Build history of the part. All positions in model axes, mm. Face numbers are marked on the shaded views. A direction names the side the tool comes from. Round coordinates to 2 decimals unless told otherwise and drop trailing zeros. Loops run counter-clockwise (first coordinate to the right, second up) from the corner with the lowest first, then second, coordinate; pieces in that order, holes last. Notation, with made-up numbers: (2, 57.25) -> (29, 57.25) arc R22 ccw to (29, 95.25) -> close; hole circle Ø6 at (47, -15). An arc over 180 degrees is marked (long way). Put each result on its own line as item: value. Start each with the question number.
Item 1: Cut at C-C, the plane x = 10. List the corners of the cut face in (y, z).
Item 2: Drill centre lines: probe 1 along Z at (x, y) = (12.5, 35.5); probe 2 along Y at (x, z) = (-8.5, 21.75); probe 3 along X at (y, z) = (84.5, 17.25). Where is each one in solid material? Low to high. Write a range as [from, to].
Item 3: Flat gauge pins, fed straight in: pin 1 Ø0.9 at (x, z) = (17.5, 11) entering from +Y; pin 2 Ø6.5 at (y, z) = (1, 9) entering from -X; pin 3 Ø12 at (x, y) = (-0.5, -0.5) entering from +Z; pin 4 Ø0.9 at (x, z) = (18, 11.5) entering from -Y. Where does each tip first touch, or does it go through?
Item 4: Cut at B-B, the plane z = 13.25. List the corners of the cut face in (x, y), plus the area to 3 significant figures.
Item 5: Pull direction Y, two halves, no side cores. Call the marked faces 1, 2, 3 and 4: +Y half, -Y half, draft (parallel to the pull), parting line (faces both ways), or undercut.
Item 6: Cut at D-D, the plane y = -48. List the corners of the cut face in (x, z), plus the area to 3 significant figures.
Item 7: Tool access for the marked faces 5 and 6: list every direction of +Z, -Z, +X, -X, +Y, -Y with a clear straight run to the whole face (end or side of a thin tool).
Item 8: Cut at A-A, the plane x = -5.5. List the corners of the cut face in (y, z).
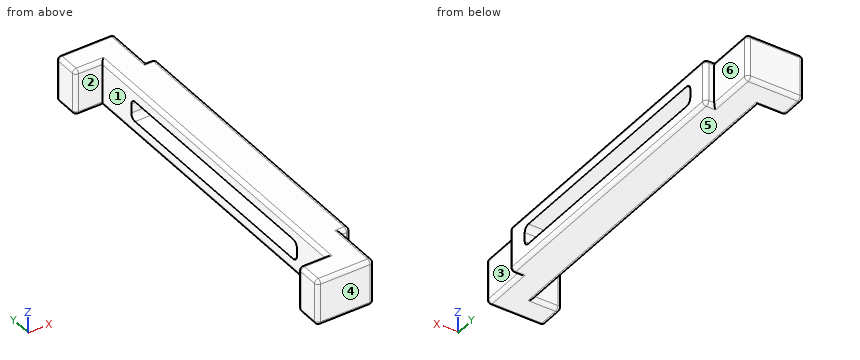
```python
from build123d import *

# Parameters (mm, degrees)
F1_DEPTH = 25
F2_R     = 2
F3_W     = 134
F3_H     = 11
F4_DEPTH = 25
F5_R     = 3
F6_R     = 2


with BuildPart() as f1:
    # F0 (on Top) → F1 (new body)
    with BuildSketch(Plane.XY):
        Polygon((-15, 90.5), (0, 90.5), (0, -90.5), (-15, -90.5), (-15, -105.5), (16, -105.5), (16, -79), (21, -79), (21, 79), (16, 79), (16, 105.5), (-15, 105.5), align=None)
    extrude(amount=F1_DEPTH)

    # F2
    f2_edges = [f1.edges().sort_by_distance(p)[0] for p in [
        (-15, -105.5, 12.5),
        (-15, 105.5, 12.5),
        (-15, 90.5, 12.5),
        (-15, -90.5, 12.5),
        (16, -105.5, 12.5),
        (21, -79, 12.5),
        (21, 79, 12.5),
        (16, 105.5, 12.5),
    ]]
    fillet(f2_edges, radius=F2_R)

    # F3 (on face) → F4 (cut)
    with BuildSketch(Plane.YZ.offset(21)):
        with Locations((0, 12.5)):
            Rectangle(F3_W, F3_H)
    extrude(amount=-F4_DEPTH, mode=Mode.SUBTRACT)

    # F5
    f5_edges = [f1.edges().sort_by_distance(p)[0] for p in [
        (10.5, -67, 7),
        (10.5, 67, 18),
        (10.5, 67, 7),
        (10.5, -67, 18),
    ]]
    fillet(f5_edges, radius=F5_R)

    # F6
    f6_edges = [f1.edges().sort_by_distance(p)[0] for p in [
        (-6.5, 90.5, 25),
        (-14.414214, 91.085786, 25),
        (0, 0, 25),
        (-15, 98, 25),
        (-6.5, -90.5, 25),
        (-14.414214, 104.914214, 25),
        (-14.414214, -91.085786, 25),
        (0.5, 105.5, 25),
        (-15, -98, 25),
        (15.414214, 104.914214, 25),
        (-14.414214, -104.914214, 25),
        (16, 91.25, 25),
        (0.5, -105.5, 25),
        (17.5, 79, 25),
        (15.414214, -104.914214, 25),
        (20.414214, 78.414214, 25),
        (16, -91.25, 25),
        (21, 0, 25),
        (17.5, -79, 25),
        (20.414214, -78.414214, 25),
        (-6.5, 90.5, 0),
        (-14.414214, 91.085786, 0),
        (0, 0, 0),
        (-15, 98, 0),
        (-6.5, -90.5, 0),
        (-14.414214, 104.914214, 0),
        (-14.414214, -91.085786, 0),
        (0.5, 105.5, 0),
        (-15, -98, 0),
        (15.414214, 104.914214, 0),
        (-14.414214, -104.914214, 0),
        (16, 91.25, 0),
        (0.5, -105.5, 0),
        (17.5, 79, 0),
        (15.414214, -104.914214, 0),
        (20.414214, 78.414214, 0),
        (16, -91.25, 0),
        (21, 0, 0),
        (17.5, -79, 0),
        (20.414214, -78.414214, 0),
    ]]
    fillet(f6_edges, radius=F6_R)


solid = f1.part
```
Reply:
1. outline: (-105.5, 2) arc R2 ccw to (-103.5, 0) -> (103.5, 0) arc R2 ccw to (105.5, 2) -> (105.5, 23) arc R2 ccw to (103.5, 25) -> (-103.5, 25) arc R2 ccw to (-105.5, 23) -> close; hole (-67, 10) arc R3 ccw to (-64, 7) -> (64, 7) arc R3 ccw to (67, 10) -> (67, 15) arc R3 ccw to (64, 18) -> (-64, 18) arc R3 ccw to (-67, 15) -> close
2. probe 1: z = [0, 7], [18, 25]
2. probe 2: y = [-105.5, -90.5], [90.5, 105.5]
2. probe 3: x = [0, 16]
3. pin 1: stops at y = 79
3. pin 2: stops at x = 0
3. pin 3: stops at z = 25
3. pin 4: stops at y = -79
4. outline: (-15, -103.5) arc R2 ccw to (-13, -105.5) -> (14, -105.5) arc R2 ccw to (16, -103.5) -> (16, -79) -> (19, -79) arc R2 ccw to (21, -77) -> (21, -67) -> (0, -67) -> (0, -90.5) -> (-13, -90.5) arc R2 ccw to (-15, -92.5) -> close; (-15, 92.5) arc R2 ccw to (-13, 90.5) -> (0, 90.5) -> (0, 67) -> (21, 67) -> (21, 77) arc R2 ccw to (19, 79) -> (16, 79) -> (16, 103.5) arc R2 ccw to (14, 105.5) -> (-13, 105.5) arc R2 ccw to (-15, 103.5) -> close
4. area: 1,800 mm^2
5. face 1: undercut
5. face 2: undercut
5. face 3: draft
5. face 4: -Y half
6. outline: (0, 2) arc R2 ccw to (2, 0) -> (19, 0) arc R2 ccw to (21, 2) -> (21, 7) -> (0, 7) -> close; (0, 18) -> (21, 18) -> (21, 23) arc R2 ccw to (19, 25) -> (2, 25) arc R2 ccw to (0, 23) -> close
6. area: 291 mm^2
7. face 5: -Z, +X, -X, +Y, -Y
7. face 6: +Z, -Z, +X, +Y
8. outline: (-105.5, 2) arc R2 ccw to (-103.5, 0) -> (-92.5, 0) arc R2 ccw to (-90.5, 2) -> (-90.5, 23) arc R2 ccw to (-92.5, 25) -> (-103.5, 25) arc R2 ccw to (-105.5, 23) -> close; (90.5, 2) arc R2 ccw to (92.5, 0) -> (103.5, 0) arc R2 ccw to (105.5, 2) -> (105.5, 23) arc R2 ccw to (103.5, 25) -> (92.5, 25) arc R2 ccw to (90.5, 23) -> close
